For this review, take the finished solid that the model builds, in its own axes (mm). A direction names the side the tool comes from. Round coordinates to 2 decimals unless told otherwise and drop trailing zeros. Write each loop counter-clockwise with the first axis right and the second up, starting at its lowest first coordinate (ties: lowest second). Pieces come first, ordered by that corner, then holes.
from build123d import *

# Parameters (mm, degrees)
SKETCH1_R           = 1.5
SKETCH1_R_2         = 4
SKETCH1_W           = 10
SKETCH1_H           = 5
BOSS_EXTRUDE1_DEPTH = 5


with BuildPart() as part:
    # Sketch1 → Boss-Extrude1 (new body)
    with BuildSketch(Plane(origin=(0, 0, 0), x_dir=(1, 0, 0), z_dir=(0, 1, 0))):
        with BuildLine():
            Line((0.102834293, -14.499635344), (22.002834293, -14.499635344))
            Line((22.002834293, -14.499635344), (22.002834293, 15.000364656))
            Line((22.002834293, 15.000364656), (64.402834293, 15.000364656))
            Line((64.402834293, 15.000364656), (64.402834293, -14.499635344))
            Line((64.402834293, -14.499635344), (90.402834293, -14.499635344))
            ThreePointArc((90.402834293, -14.499635344), (100.683758076, -7.411489913), (97.715103143, 4.718072625))
            Line((97.715103143, 4.718072625), (57.168590047, 40.797111428))
            ThreePointArc((57.168590047, 40.797111428), (52.935602616, 42.969014799), (48.180396076, 42.816182826))
            Line((48.180396076, 42.816182826), (-8.032001051, 26.333549436))
            ThreePointArc((-8.032001051, 26.333549436), (-12.703498591, 23.092010868), (-14.499635344, 17.697165707))
            Line((-14.499635344, 17.697165707), (-14.499635344, -0.102834293))
            ThreePointArc((-14.499635344, -0.102834293), (-10.18007565, -10.325505303), (0.102834293, -14.499635344))
        make_face()
        Circle(SKETCH1_R, mode=Mode.SUBTRACT)
        with Locations((90.402834293, -3.499635344)):
            Circle(SKETCH1_R_2, mode=Mode.SUBTRACT)
        with Locations((50.853448768, 33.7)):
            Circle(SKETCH1_R, mode=Mode.SUBTRACT)
        with Locations((10.7, -9.999635344)):
            Rectangle(SKETCH1_W, SKETCH1_H, mode=Mode.SUBTRACT)
        with Locations((75.602834293, -9.999635344)):
            Rectangle(SKETCH1_W, SKETCH1_H, mode=Mode.SUBTRACT)
    extrude(amount=BOSS_EXTRUDE1_DEPTH)


solid = part.part
(1) For faces 1 (the face through (100.62, 2.46, 7.58)), 2 (the face through (5.7, 2, 10)), 3 (the face through (22.003, 2, 0)), list the 3-axis set-ups (+Z, -Z, +X, -X, +Y, -Y) from which the entire face can be reached by the end or side of a thin tool; tool diameter is ignored.
Geometry check:
face 1: +X, +Y, -Y
face 2: +Y, -Y
face 3: +Z, +Y, -Y
(2) We need section A-A, the plane x = 72.5. Give the boundary of the cut face in (y, z).
Geometry check:
outline: (0, -27.15) - (5, -27.15) - (5, 7.5) - (0, 7.5) - close; (0, 12.5) - (5, 12.5) - (5, 14.5) - (0, 14.5) - close
(3) For line 1 along X through (y, z) = (1.35, 0); line 2 along X through (y, z) = (0.9, 2); line 3 along X through (y, z) = (1.1, 12), list the stretches that pass through material, from the lowest coordinate up.
Geometry check:
line 1: x = -14.5 to -1.5, 1.5 to 22, 64.4 to 88.47, 92.34 to 100.83
line 2: x = -14.36 to 22, 64.4 to 86.69, 94.11 to 101.3
line 3: x = -8.14 to 5.7, 15.7 to 22, 64.4 to 70.6, 80.6 to 97.38
(4) We need section B-B, the plane y = 1.4. Give the boundary of the cut face in (x, z).
Geometry check:
outline: (-14.5, -17.7) arc R9 ccw to (-8.03, -26.33) - (48.18, -42.82) arc R9.5 ccw to (57.17, -40.8) - (97.72, -4.72) arc R11 ccw to (90.4, 14.5) - (64.4, 14.5) - (64.4, -15) - (22, -15) - (22, 14.5) - (0.1, 14.5) arc R14.5 ccw to (-14.5, 0.1) - close; hole circle Ø3 at (0, 0); hole (5.7, 7.5) - (15.7, 7.5) - (15.7, 12.5) - (5.7, 12.5) - close; hole circle Ø3 at (50.85, -33.7); hole (70.6, 7.5) - (80.6, 7.5) - (80.6, 12.5) - (70.6, 12.5) - close; hole circle Ø8 at (90.4, 3.5)
(5) Mouldability with a two-part tool opening along X and no side actions: class faces 4 (the face through (-12.65, 2.46, -23.16)), 5 (the face through (43, 5, -21)), 6 (the face through (53.001, 2.465, -42.954)), 7 (the face through (70.603, 2, 10)) as pulls with the +X half, pulls with the -X half, needs draft (parallel to the pull), parting line crosses it, or undercut.
Geometry check:
face 4: pulls with the -X half
face 5: needs draft
face 6: parting line crosses it
face 7: undercut
(6) We need section C-C, the plane z = -33.7. Give the boundary of the cut face in (x, y).
Geometry check:
outline: (17.09, 0) - (49.35, 0) - (49.35, 5) - (17.09, 5) - close; (52.35, 0) - (65.14, 0) - (65.14, 5) - (52.35, 5) - close
(7) For pin 1 Ø1.5 at (y, z) = (1.5, -3) entering from +X; pin 2 Ø2.5 at (x, z) = (50.85, -33.7) entering from -Y; pin 3 Ø1.5 at (x, y) = (76, 1.5) entering from -Z; pin 4 Ø1.5 at (y, z) = (2.5, 11) entering from +X, all flat-tipped, find the tip position at first contact; note any pin that passes through.
Geometry check:
pin 1: stops at x = 99.78
pin 2: passes through
pin 3: stops at z = -24.71
pin 4: stops at x = 99.09
(8) We need section D-D, the plane x = 38. Give the boundary of the cut face in (y, z), and give its area (3 significant figures).
Geometry check:
outline: (0, -39.83) - (5, -39.83) - (5, -15) - (0, -15) - close
area: 124 mm2
